Design review of the part built by this model. Coordinates are the model's own, in mm. Face numbers are marked on the shaded views. A direction names the side the tool comes from. Coordinates: 2 decimals unless noted, no trailing zeros. Write each loop counter-clockwise with the first axis right and the second up, starting at its lowest first coordinate (ties: lowest second). Pieces come first, ordered by that corner, then holes. Notation, with made-up numbers: (0, -30) -> (30, -30) arc R28 cw to (30, -6) -> close; hole circle Ø6 at (-6.5, -11). An arc over 180 degrees is marked (long way). Answer in a Markdown table with one row per item. Add a question column.
Item 1: Draft analysis for pull direction X (two halves, no side actions). For the marked faces 3 and 4, state which applies: released by +X, released by -X, zero draft, split by the parting line, or undercut.
Item 2: Take a section at D-D, the plane x = -2. Write out the cut boundary in (y, z).
Item 3: To check wall thickness, follow line 1 (X direction, y = 0.8, z = -5); line 2 (X direction, y = 1.25, z = 6.5); line 3 (Y direction, x = 11.5, z = 0). State the ranges of each line that lie inside material, in increasing order.
Item 4: For the marked faces 1 and 2, list the 3-axis set-ups (+Z, -Z, +X, -X, +Y, -Y) from which the entire face can be reached by the end or side of a thin tool; tool diameter is ignored.
Item 5: Clearance check with flat-ended pins moving along their axes: P1, Ø1.5, axis at y = -2.5, z = 2, coming from the -X side; P2, Ø4, axis at x = 0.5, y = -3.5, coming from the +Z side; P3, Ø6, axis at y = -4, z = -3.5, coming from the +X side; P4, Ø5, axis at x = 4, z = 1.5, coming from the -Y side. State where each tip first meets the part, or that it passes through.
Item 6: Take a section at A-A, the plane z = 7.5. Write out the cut boundary in (x, y), and give its area (3 significant figures).
Item 7: Take a section at B-B, the plane x = 7.1. Write out the cut boundary in (y, z), and give its area (3 significant figures).
Item 8: Take a section at C-C, the plane y = 2. Write out the cut boundary in (x, z), and give its area (3 significant figures).
from build123d import *

# Parameters (mm, degrees)
SKETCH_1_R      = 1.75
SKETCH_1_R_2    = 1.45
EXTRUDE_1_DEPTH = 3
FILLET_1_R      = 3
EXTRUDE_2_DEPTH = 2.5
FILLET_2_R      = 1.5
FILLET_3_R      = 1


with BuildPart() as part:
    # 草图1 → 凸台-拉伸1 (new body)
    with BuildSketch(Plane(origin=(0, 0, 0), x_dir=(1, 0, 0), z_dir=(0, 1, 0))):
        Polygon((-13, 22.5), (-13, -12.5), (13, -12.5), (13, 22.5), (13, 26.25), (-13, 26.25), align=None)
        with Locations(Location((-10, -7.5, 0), (0, 0, 270))):
            Circle(SKETCH_1_R, mode=Mode.SUBTRACT)
        with Locations(Location((10, -7.5, 0), (0, 0, 270))):
            Circle(SKETCH_1_R, mode=Mode.SUBTRACT)
        with Locations(Location((0, 23.25, 0), (0, 0, 270))):
            Circle(SKETCH_1_R_2, mode=Mode.SUBTRACT)
        with Locations(Location((-7.1, 5, 0), (0, 0, 270))):
            Circle(SKETCH_1_R_2, mode=Mode.SUBTRACT)
        with Locations(Location((7.1, 5, 0), (0, 0, 270))):
            Circle(SKETCH_1_R_2, mode=Mode.SUBTRACT)
    extrude(amount=EXTRUDE_1_DEPTH)

    # 圆角1
    fillet_1_edges = [part.edges().sort_by_distance(p)[0] for p in [
        (13, 1.5, 12.5),
        (-13, 1.5, 12.5),
        (-13, 1.5, -26.25),
        (13, 1.5, -26.25),
    ]]
    fillet(fillet_1_edges, radius=FILLET_1_R)

    # 草图3 → 凸台-拉伸2 (add, symmetric)
    with BuildSketch(Plane(origin=(0, 0, 0), x_dir=(0, 0, -1), z_dir=(1, 0, 0))):
        Polygon((0, 0), (0, -10), (15.25, 0), align=None)
    extrude(amount=EXTRUDE_2_DEPTH, both=True)

    # 圆角2
    fillet_2_edges = [part.edges().sort_by_distance(p)[0] for p in [
        (-2.5, 0, -7.625),
        (0, 0, -15.25),
        (2.5, 0, -7.625),
    ]]
    fillet(fillet_2_edges, radius=FILLET_2_R)

    # 圆角3
    fillet_3_edges = [part.edges().sort_by_distance(p)[0] for p in [
        (0, -10, 0),
    ]]
    fillet(fillet_3_edges, radius=FILLET_3_R)


solid = part.part
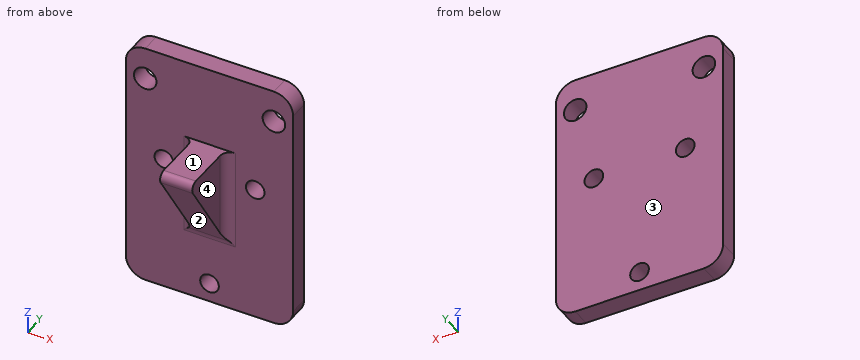
Answers:
| question | item | result |
|---|---|---|
| 1 | face 3 | zero draft |
| 1 | face 4 | released by +X |
| 2 | outline | (-8.98, -1.55) -> (-0.25, -14.88) arc R1.5 cw to (0, -15.7) -> (0, -26.25) -> (3, -26.25) -> (3, 12.5) -> (0, 12.5) -> (0, 0) -> (-8.15, 0) arc R1 ccw to start |
| 3 | line 1 | x = -13 to -8.55, -5.65 to 5.65, 8.55 to 13 |
| 3 | line 2 | x = -13 to -11.44, -8.56 to 8.56, 11.44 to 13 |
| 3 | line 3 | y = 0 to 3 |
| 4 | face 1 | +Z, +X, -X, -Y |
| 4 | face 2 | -Z, +X, -X, -Y |
| 5 | P1 | passes through |
| 5 | P2 | stops at z = 0 |
| 5 | P3 | stops at x = 2.59 |
| 5 | P4 | stops at y = -9.01 |
| 6 | outline | (-13, 0) -> (-11.75, 0) -> (-11.75, 3) -> (-13, 3) -> close; (-8.25, 0) -> (8.25, 0) -> (8.25, 3) -> (-8.25, 3) -> close; (11.75, 0) -> (13, 0) -> (13, 3) -> (11.75, 3) -> close |
| 6 | area | 57.0 mm^2 |
| 7 | outline | (0, -26.25) -> (3, -26.25) -> (3, -6.45) -> (0, -6.45) -> close; (0, -3.55) -> (3, -3.55) -> (3, 12.5) -> (0, 12.5) -> close |
| 7 | area | 108 mm^2 |
| 8 | outline | (-13, -23.25) arc R3 ccw to (-10, -26.25) -> (10, -26.25) arc R3 ccw to (13, -23.25) -> (13, 9.5) arc R3 ccw to (10, 12.5) -> (-10, 12.5) arc R3 ccw to (-13, 9.5) -> close; hole circle Ø3.5 at (-10, 7.5); hole circle Ø2.9 at (-7.1, -5); hole circle Ø2.9 at (0, -23.25); hole circle Ø2.9 at (7.1, -5); hole circle Ø3.5 at (10, 7.5) |
| 8 | area | 961 mm^2 |
